Here's how the part is built. I have some questions about the finished solid (model axes, mm). A direction names the side the tool comes from. Round coordinates to 2 decimals unless told otherwise and drop trailing zeros. Loops run counter-clockwise (first coordinate to the right, second up) from the corner with the lowest first, then second, coordinate; pieces in that order, holes last. Notation, with made-up numbers: (68.5, 21) - (92.5, 21) arc R26 cw to (92.5, 50) - close; hole circle Ø2 at (1, -3.75). An arc over 180 degrees is marked (long way). Return JSON: item names as keys, results as strings. Group by question number.
```python
from build123d import *

# Parameters (mm, degrees)
SKIZZE1_W                       = 25
SKIZZE1_H                       = 16
AUFSATZ_LINEAR_AUSTRAGEN1_DEPTH = 13
SKIZZE2_W                       = 25
SKIZZE2_H                       = 7.5
SCHNITT_LINEAR_AUSTRAGEN1_DEPTH = 5
SKIZZE3_W                       = 6
SKIZZE3_H                       = 16
AUFSATZ_LINEAR_AUSTRAGEN2_DEPTH = 5.4
VERRUNDUNG1_R                   = 1
FASE1_SIZE                      = 0.5
VERRUNDUNG2_R                   = 4
VERRUNDUNG3_R                   = 1


with BuildPart() as part:
    # Skizze1 → Aufsatz-Linear austragen1 (new body)
    with BuildSketch(Plane(origin=(0, 0, 0), x_dir=(1, 0, 0), z_dir=(0, 1, 0))):
        Rectangle(SKIZZE1_W, SKIZZE1_H)
    extrude(amount=AUFSATZ_LINEAR_AUSTRAGEN1_DEPTH)

    # Skizze2 → Schnitt-Linear austragen1 (cut)
    with BuildSketch(Plane(origin=(0, 13, 0), x_dir=(1, 0, 0), z_dir=(0, 1, 0))):
        Rectangle(SKIZZE2_W, SKIZZE2_H)
    extrude(amount=-SCHNITT_LINEAR_AUSTRAGEN1_DEPTH, mode=Mode.SUBTRACT)

    # Skizze3 → Aufsatz-Linear austragen2 (add)
    with BuildSketch(Plane.XZ):
        Rectangle(SKIZZE3_W, SKIZZE3_H)
    extrude(amount=AUFSATZ_LINEAR_AUSTRAGEN2_DEPTH)

    # Verrundung1
    verrundung1_edges = [part.edges().sort_by_distance(p)[0] for p in [
        (12.5, 10.5, -3.75),
        (12.5, 10.5, 3.75),
        (-12.5, 10.5, 3.75),
        (-12.5, 10.5, -3.75),
        (0, 13, -3.75),
        (0, 13, 3.75),
    ]]
    fillet(verrundung1_edges, radius=VERRUNDUNG1_R)

    # Fase1
    fase1_edges = [part.edges().sort_by_distance(p)[0] for p in [
        (7.75, 0, 8),
        (-7.75, 0, -8),
        (3, 0, 0),
        (3, -2.7, -8),
        (3, -2.7, 8),
        (-3, 0, 0),
        (-3, -2.7, 8),
        (-3, -2.7, -8),
        (3, -5.4, 0),
        (-3, -5.4, 0),
        (-7.75, 0, 8),
        (-12.5, 0, 0),
        (7.75, 0, -8),
        (12.5, 0, 0),
    ]]
    chamfer(fase1_edges, length=FASE1_SIZE)

    # Verrundung2
    verrundung2_edges = [part.edges().sort_by_distance(p)[0] for p in [
        (12.5, 8, 0),
        (-12.5, 8, 0),
    ]]
    fillet(verrundung2_edges, radius=VERRUNDUNG2_R)

    # Verrundung3
    # the kernel refuses this fillet: 1 mm, written as the material it takes off along each edge
    with BuildSketch(Plane(origin=(-11.5, 12, 4.75), x_dir=(0, 1, 0), z_dir=(-1, 0, 0))) as verrundung3_piece_1_section:
        Polygon((0, 0), (VERRUNDUNG3_R, 0), (VERRUNDUNG3_R, VERRUNDUNG3_R), (0, VERRUNDUNG3_R), align=None)
    verrundung3_piece_1 = extrude(amount=VERRUNDUNG3_R, mode=Mode.PRIVATE)
    verrundung3_piece_1 = verrundung3_piece_1 - Plane(origin=(-11.5, 12, 4.75), x_dir=(0, -0.7071067811865475, 0.7071067811865475), z_dir=(-1, 0, 0)) * Sphere(VERRUNDUNG3_R, mode=Mode.PRIVATE)
    add(verrundung3_piece_1, mode=Mode.SUBTRACT)
    with BuildSketch(Plane(origin=(11.5, 12, 4.75), x_dir=(1, 0, 0), z_dir=(0, 1, 0))) as verrundung3_piece_2_section:
        Polygon((0, 0), (VERRUNDUNG3_R, 0), (VERRUNDUNG3_R, VERRUNDUNG3_R), (0, VERRUNDUNG3_R), align=None)
    verrundung3_piece_2 = extrude(amount=VERRUNDUNG3_R, mode=Mode.PRIVATE)
    verrundung3_piece_2 = verrundung3_piece_2 - Plane(origin=(11.5, 12, 4.75), x_dir=(-0.7071067811865475, 0, 0.7071067811865475), z_dir=(0, 1, 0)) * Sphere(VERRUNDUNG3_R, mode=Mode.PRIVATE)
    add(verrundung3_piece_2, mode=Mode.SUBTRACT)
    with BuildSketch(Plane(origin=(-11.5, 12, -4.75), x_dir=(0, 1, 0), z_dir=(-1, 0, 0))) as verrundung3_piece_3_section:
        Polygon((0, 0), (VERRUNDUNG3_R, 0), (VERRUNDUNG3_R, -VERRUNDUNG3_R), (0, -VERRUNDUNG3_R), align=None)
    verrundung3_piece_3 = extrude(amount=VERRUNDUNG3_R, mode=Mode.PRIVATE)
    verrundung3_piece_3 = verrundung3_piece_3 - Plane(origin=(-11.5, 12, -4.75), x_dir=(0, -0.7071067811865475, -0.7071067811865475), z_dir=(-1, 0, 0)) * Sphere(VERRUNDUNG3_R, mode=Mode.PRIVATE)
    add(verrundung3_piece_3, mode=Mode.SUBTRACT)
    with BuildSketch(Plane(origin=(11.5, 12, -4.75), x_dir=(1, 0, 0), z_dir=(0, 1, 0))) as verrundung3_piece_4_section:
        Polygon((0, 0), (VERRUNDUNG3_R, 0), (VERRUNDUNG3_R, -VERRUNDUNG3_R), (0, -VERRUNDUNG3_R), align=None)
    verrundung3_piece_4 = extrude(amount=VERRUNDUNG3_R, mode=Mode.PRIVATE)
    verrundung3_piece_4 = verrundung3_piece_4 - Plane(origin=(11.5, 12, -4.75), x_dir=(-0.7071067811865475, 0, -0.7071067811865475), z_dir=(0, 1, 0)) * Sphere(VERRUNDUNG3_R, mode=Mode.PRIVATE)
    add(verrundung3_piece_4, mode=Mode.SUBTRACT)
    with BuildSketch(Plane(origin=(-11.5, 12, -7), x_dir=(0, 0, -1), z_dir=(-1, 0, 0))) as verrundung3_piece_5_section:
        Polygon((0, 0), (VERRUNDUNG3_R, 0), (VERRUNDUNG3_R, -VERRUNDUNG3_R), (0, -VERRUNDUNG3_R), align=None)
    verrundung3_piece_5 = extrude(amount=VERRUNDUNG3_R, mode=Mode.PRIVATE)
    verrundung3_piece_5 = verrundung3_piece_5 - Plane(origin=(-11.5, 12, -7), x_dir=(0, -0.7071067811865475, 0.7071067811865475), z_dir=(-1, 0, 0)) * Sphere(VERRUNDUNG3_R, mode=Mode.PRIVATE)
    add(verrundung3_piece_5, mode=Mode.SUBTRACT)
    with BuildSketch(Plane(origin=(-11.5, 12, 7), x_dir=(0, 1, 0), z_dir=(-1, 0, 0))) as verrundung3_piece_6_section:
        Polygon((0, 0), (VERRUNDUNG3_R, 0), (VERRUNDUNG3_R, -VERRUNDUNG3_R), (0, -VERRUNDUNG3_R), align=None)
    verrundung3_piece_6 = extrude(amount=VERRUNDUNG3_R, mode=Mode.PRIVATE)
    verrundung3_piece_6 = verrundung3_piece_6 - Plane(origin=(-11.5, 12, 7), x_dir=(0, -0.7071067811865475, -0.7071067811865475), z_dir=(-1, 0, 0)) * Sphere(VERRUNDUNG3_R, mode=Mode.PRIVATE)
    add(verrundung3_piece_6, mode=Mode.SUBTRACT)
    with BuildSketch(Plane(origin=(11.5, 12, 7), x_dir=(0, 1, 0), z_dir=(1, 0, 0))) as verrundung3_piece_7_section:
        Polygon((0, 0), (VERRUNDUNG3_R, 0), (VERRUNDUNG3_R, VERRUNDUNG3_R), (0, VERRUNDUNG3_R), align=None)
    verrundung3_piece_7 = extrude(amount=VERRUNDUNG3_R, mode=Mode.PRIVATE)
    verrundung3_piece_7 = verrundung3_piece_7 - Plane(origin=(11.5, 12, 7), x_dir=(0, -0.7071067811865475, -0.7071067811865475), z_dir=(1, 0, 0)) * Sphere(VERRUNDUNG3_R, mode=Mode.PRIVATE)
    add(verrundung3_piece_7, mode=Mode.SUBTRACT)
    with BuildSketch(Plane(origin=(11.5, 12, -7), x_dir=(1, 0, 0), z_dir=(0, 0, -1))) as verrundung3_piece_8_section:
        Polygon((0, 0), (VERRUNDUNG3_R, 0), (VERRUNDUNG3_R, -VERRUNDUNG3_R), (0, -VERRUNDUNG3_R), align=None)
    verrundung3_piece_8 = extrude(amount=VERRUNDUNG3_R, mode=Mode.PRIVATE)
    verrundung3_piece_8 = verrundung3_piece_8 - Plane(origin=(11.5, 12, -7), x_dir=(-0.7071067811865475, -0.7071067811865475, 0), z_dir=(0, 0, -1)) * Sphere(VERRUNDUNG3_R, mode=Mode.PRIVATE)
    add(verrundung3_piece_8, mode=Mode.SUBTRACT)
    with BuildSketch(Plane(origin=(-12.5, 13, -7), x_dir=(0, -1, 0), z_dir=(0, 0, 1)), Plane(origin=(-12.5, 13, 4.75), x_dir=(0, -1, 0), z_dir=(0, 0, 1))) as verrundung3_piece_9:
        with BuildLine():
            CenterArc((VERRUNDUNG3_R, VERRUNDUNG3_R), VERRUNDUNG3_R, 180, 90)
            Line((0, VERRUNDUNG3_R), (0, 0))
            Line((0, 0), (VERRUNDUNG3_R, 0))
        make_face()
    extrude(amount=2.25, mode=Mode.SUBTRACT)
    with BuildSketch(Plane(origin=(-11.5, 13, 8), x_dir=(0, 0, -1), z_dir=(1, 0, 0)), Plane(origin=(11.5, 13, -8), x_dir=(0, 0, 1), z_dir=(-1, 0, 0))) as verrundung3_piece_10:
        with BuildLine():
            CenterArc((VERRUNDUNG3_R, -VERRUNDUNG3_R), VERRUNDUNG3_R, 90, 90)
            Line((0, -VERRUNDUNG3_R), (0, 0))
            Line((0, 0), (VERRUNDUNG3_R, 0))
        make_face()
    extrude(amount=23, mode=Mode.SUBTRACT)
    with BuildSketch(Plane(origin=(12.5, 13, 7), x_dir=(-1, 0, 0), z_dir=(0, 0, -1)), Plane(origin=(12.5, 13, -4.75), x_dir=(-1, 0, 0), z_dir=(0, 0, -1))) as verrundung3_piece_11:
        with BuildLine():
            CenterArc((VERRUNDUNG3_R, -VERRUNDUNG3_R), VERRUNDUNG3_R, 90, 90)
            Line((0, -VERRUNDUNG3_R), (0, 0))
            Line((0, 0), (VERRUNDUNG3_R, 0))
        make_face()
    extrude(amount=2.25, mode=Mode.SUBTRACT)
    with BuildSketch(Plane(origin=(12.5, -2, 8), x_dir=(-1, 0, 0), z_dir=(0, 1, 0)), Plane(origin=(-12.5, -2, 8), x_dir=(0, 0, -1), z_dir=(0, 1, 0))) as verrundung3_piece_12:
        with BuildLine():
            CenterArc((VERRUNDUNG3_R, -VERRUNDUNG3_R), VERRUNDUNG3_R, 90, 90)
            Line((0, -VERRUNDUNG3_R), (0, 0))
            Line((0, 0), (VERRUNDUNG3_R, 0))
        make_face()
    extrude(amount=14, mode=Mode.SUBTRACT)
    with BuildSketch(Plane(origin=(-12.5, -2, -8), x_dir=(0, 0, 1), z_dir=(0, 1, 0)), Plane(origin=(12.5, -2, -8), x_dir=(-1, 0, 0), z_dir=(0, 1, 0))) as verrundung3_piece_13:
        with BuildLine():
            CenterArc((VERRUNDUNG3_R, VERRUNDUNG3_R), VERRUNDUNG3_R, 180, 90)
            Line((0, VERRUNDUNG3_R), (0, 0))
            Line((0, 0), (VERRUNDUNG3_R, 0))
        make_face()
    extrude(amount=14, mode=Mode.SUBTRACT)


solid = part.part
```
Q1. If we mould it in two halves opening along Z, with no side actions, what happens to faces 1 (the cylindrical face through (-12.215, 6.021, 7.699)), 2 (the flat face through (8, 0, 0)), 3 (the flat face through (0, 8, 0))? For each: +Z half, -Z half, draft (parallel to the pull), parting line (faces both ways), or undercut.
Q2. For faces 4 (the cylindrical face through (-12.215, 8.833, 4.051)), 5 (the flat face through (-3, -3, 0)), 6 (the flat face through (3, -3, 0)), which set-ups out of +Z, -Z, +X, -X, +Y, -Y let a thin tool reach every point of the face, with its end or its side?
Q3. Imagine slicing it at B-B, the plane z = -3.25. List the corners of the cut face in (x, y) for me.
Q4. Imagine slicing it at D-D, the plane y = -2.75. List the corners of the cut face in (x, z) for me, and give its area (3 significant figures).
Q5. Imagine slicing it at A-A, the plane y = 11.25. List the corners of the cut face in (x, z) for me, and give its area (3 significant figures).
Q6. Please list where these lines run through material, in increasing order: line 1 (Z direction, x = -5, y = 11.5); line 2 (Y direction, x = -6, z = -1.5); line 3 (X direction, y = -4.5, z = 6.25).
Q7. Imagine slicing it at C-C, the plane x = -1.25. List the corners of the cut face in (y, z) for me, and give its area (3 significant figures).
Q8. Will these pins go through, and if not, where does the flat tip stop? pin 1 Ø2.5 at (x, z) = (8.5, 0) entering from -Y; pin 2 Ø3 at (x, z) = (9, -2) entering from +Y; pin 3 Ø5 at (y, z) = (-3.5, -2.5) entering from -X.
Output values:
{
 "1": {"face 1": "+Z half", "face 2": "draft", "face 3": "undercut"},
 "2": {"face 4": "-X, +Y", "face 5": "+Z, -Z, -X, -Y", "face 6": "+Z, -Z, +X, -Y"},
 "3": {"outline": "(-12.5, 0.5) - (-12, 0) - (-3.5, 0) - (-3, -0.5) - (-3, -4.9) - (-2.5, -5.4) - (2.5, -5.4) - (3, -4.9) - (3, -0.5) - (3.5, 0) - (12, 0) - (12.5, 0.5) - (12.5, 4) arc R4 ccw to (8.5, 8) - (-8.5, 8) arc R4 ccw to (-12.5, 4) - close"},
 "4": {"outline": "(-3, -7.5) - (-2.5, -8) - (2.5, -8) - (3, -7.5) - (3, 7.5) - (2.5, 8) - (-2.5, 8) - (-3, 7.5) - close", "area": "95.5 mm^2"},
 "5": {"outline": "(-12.5, -7) arc R1 ccw to (-11.5, -8) - (11.5, -8) arc R1 ccw to (12.5, -7) - (12.5, -4.75) arc R1 ccw to (11.5, -3.75) - (-11.5, -3.75) arc R1 ccw to (-12.5, -4.75) - close; (-12.5, 4.75) arc R1 ccw to (-11.5, 3.75) - (11.5, 3.75) arc R1 ccw to (12.5, 4.75) - (12.5, 7) arc R1 ccw to (11.5, 8) - (-11.5, 8) arc R1 ccw to (-12.5, 7) - close", "area": "211 mm^2"},
 "6": {"line 1": "z = -8 to -3.75, 3.75 to 8", "line 2": "y = 0 to 8", "line 3": "x = -3 to 3"},
 "7": {"outline": "(-5.4, -8) - (12, -8) arc R1 ccw to (13, -7) - (13, -4.75) arc R1 ccw to (12, -3.75) - (8, -3.75) - (8, 3.75) - (12, 3.75) arc R1 ccw to (13, 4.75) - (13, 7) arc R1 ccw to (12, 8) - (-5.4, 8) - close", "area": "256 mm^2"},
 "8": {"pin 1": "stops at y = 0", "pin 2": "stops at y = 8", "pin 3": "stops at x = -3"}
}
